Geometry: final body of the model. Coordinates: model frame, mm. A direction names the side the tool comes from. Coordinates: 2 decimals unless noted, no trailing zeros. Order: outer loops, then holes, each group sorted by start corner. A loop starts at its lowest first (then second) coordinate and runs counter-clockwise, first axis right, second up. Notation, with made-up numbers: (10, 59.5) -> (20, 59.5) arc R31 ccw to (20, 86.5) -> close; hole circle Ø8 at (11.25, 37). An arc over 180 degrees is marked (long way). Answer in a Markdown table with one row per item. Add a question column.
1) Set-up query: faces 4 (the face through (1.2, 14, 11)), 5 (the face through (0, 14, 5)), 6 (the face through (56.9, 14, 5)). Return all of +Z, -Z, +X, -X, +Y, -Y with unobstructed straight access to the full face (end or side cutting, diameter ignored); none if empty.
2) Pull-direction query (X, two-part tool) for faces 1 (the face through (57.3, 14, 11)), 2 (the face through (29, 27.9, 17)), 3 (the face through (29, 1.2, 11)); classes: +X half, -X half, draft (parallel to the pull), parting line (faces both ways), or undercut.
3) Section query C-C on y = 8.5. Return the cut outline in (x, z).
4) Ray query, line 1 (X direction, y = 6.25, z = 6); line 2 (Y direction, x = 8.5, z = 16); line 3 (Y direction, x = 23.5, z = 11.5). Return the intervals inside material, ascending. Write a range as from..to.
5) Section query B-B on z = 2. Return the cut outline in (x, y).
6) Section query A-A on x = 31. Return the cut outline in (y, z).
7) Contact query for flat-ended pins moving along their axis: P1, Ø8, axis at x = 24, z = 16.5, coming from the +Y side; P2, Ø3, axis at y = 11.5, z = 6.5, coming from the -X side; P3, Ø2, axis at x = 30.5, z = 14, coming from the -Y side. Output: stop coordinate, or through.
Autodesk Inventor part; units mm, degrees
ref_plane "YZ Plane" through (0, 0, 0) normal (1, 0, 0) x (0, 1, 0)
ref_plane "XZ Plane" through (0, 0, 0) normal (0, 1, 0) x (-1, 0, 0)
ref_plane "XY Plane" through (0, 0, 0) normal (0, 0, 1) x (1, 0, 0)
sketch "Sketch1" plane through (0, 0, 0) normal (0, 0, 1) x (1, 0, 0)
  line L0 (0, 0) -> (56.9, 0)
  line L1 (56.9, 0) -> (56.9, 27.9)
  line L2 (56.9, 27.9) -> (0, 27.9)
  line L3 (0, 27.9) -> (0, 0)
  line L4 (1.2, 26.7) -> (55.7, 26.7)
  line L5 (55.7, 26.7) -> (55.7, 1.2)
  line L6 (55.7, 1.2) -> (1.2, 1.2)
  line L7 (1.2, 1.2) -> (1.2, 26.7)
  dimension "d0" = 56.9
  dimension "d1" = 27.9
  dimension "d2" = 1.2
  dimension "d3" = 1.2
  dimension "d4" = 1.2
  dimension "d5" = 1.2
extrude "Extrusion1" add sketch "Sketch1" along normal blind 10
sketch "Sketch3" plane through (0, 0, 10) normal (0, 0, 1) x (1, 0, 0)
  line L0 (1.2, 26.7) -> (55.7, 26.7)
  line L1 (55.7, 26.7) -> (55.7, 1.2)
  line L2 (1.2, 26.7) -> (55.7, 26.7)
  line L3 (55.7, 26.7) -> (55.7, 1.2)
  line L4 (55.7, 1.2) -> (1.2, 1.2)
  line L5 (1.2, 1.2) -> (1.2, 26.7)
  line L6 (-0.4, 28.3) -> (57.3, 28.3)
  line L7 (57.3, 28.3) -> (57.3, -0.4)
  line L8 (57.3, -0.4) -> (-0.4, -0.4)
  line L9 (-0.4, -0.4) -> (-0.4, 28.3)
  point P0 (0, 0)
  dimension "d8" = 1.6
  dimension "d9" = 1.6
  dimension "d10" = 1.6
  dimension "d11" = 1.6
extrude "Extrusion2" add sketch "Sketch3" along normal blind 2
sketch "Sketch4" plane through (0, 0, 12) normal (0, 0, 1) x (1, 0, 0)
  line L0 (1.2, 26.7) -> (55.7, 26.7)
  line L1 (55.7, 26.7) -> (55.7, 1.2)
  line L2 (1.2, 26.7) -> (55.7, 26.7)
  line L3 (55.7, 26.7) -> (55.7, 1.2)
  line L4 (55.7, 1.2) -> (1.2, 1.2)
  line L5 (1.2, 1.2) -> (1.2, 26.7)
  line L6 (56.9, 27.9) -> (0, 27.9)
  line L7 (56.9, 0) -> (56.9, 27.9)
  line L8 (0, 27.9) -> (56.9, 27.9)
  line L9 (56.9, 27.9) -> (56.9, 0)
  line L10 (56.9, 0) -> (0, 0)
  line L11 (0, 0) -> (0, 27.9)
extrude "Extrusion3" add sketch "Sketch4" along normal blind 10
properties part number "Connector"
Result:
| question | item | result |
|---|---|---|
| 1 | face 4 | +Z, -Z |
| 1 | face 5 | -Z, -X, +Y, -Y |
| 1 | face 6 | -Z, +X, +Y, -Y |
| 2 | face 1 | +X half |
| 2 | face 2 | draft |
| 2 | face 3 | undercut |
| 3 | outline | (-0.4, 10) -> (0, 10) -> (0, 0) -> (1.2, 0) -> (1.2, 22) -> (0, 22) -> (0, 12) -> (-0.4, 12) -> close; (55.7, 0) -> (56.9, 0) -> (56.9, 10) -> (57.3, 10) -> (57.3, 12) -> (56.9, 12) -> (56.9, 22) -> (55.7, 22) -> close |
| 4 | line 1 | 0..1.2, 55.7..56.9 |
| 4 | line 2 | 0..1.2, 26.7..27.9 |
| 4 | line 3 | -0.4..1.2, 26.7..28.3 |
| 5 | outline | (0, 0) -> (56.9, 0) -> (56.9, 27.9) -> (0, 27.9) -> close; hole (1.2, 1.2) -> (55.7, 1.2) -> (55.7, 26.7) -> (1.2, 26.7) -> close |
| 6 | outline | (-0.4, 10) -> (0, 10) -> (0, 0) -> (1.2, 0) -> (1.2, 22) -> (0, 22) -> (0, 12) -> (-0.4, 12) -> close; (26.7, 0) -> (27.9, 0) -> (27.9, 10) -> (28.3, 10) -> (28.3, 12) -> (27.9, 12) -> (27.9, 22) -> (26.7, 22) -> close |
| 7 | P1 | y = 27.9 |
| 7 | P2 | x = 0 |
| 7 | P3 | y = 0 |
